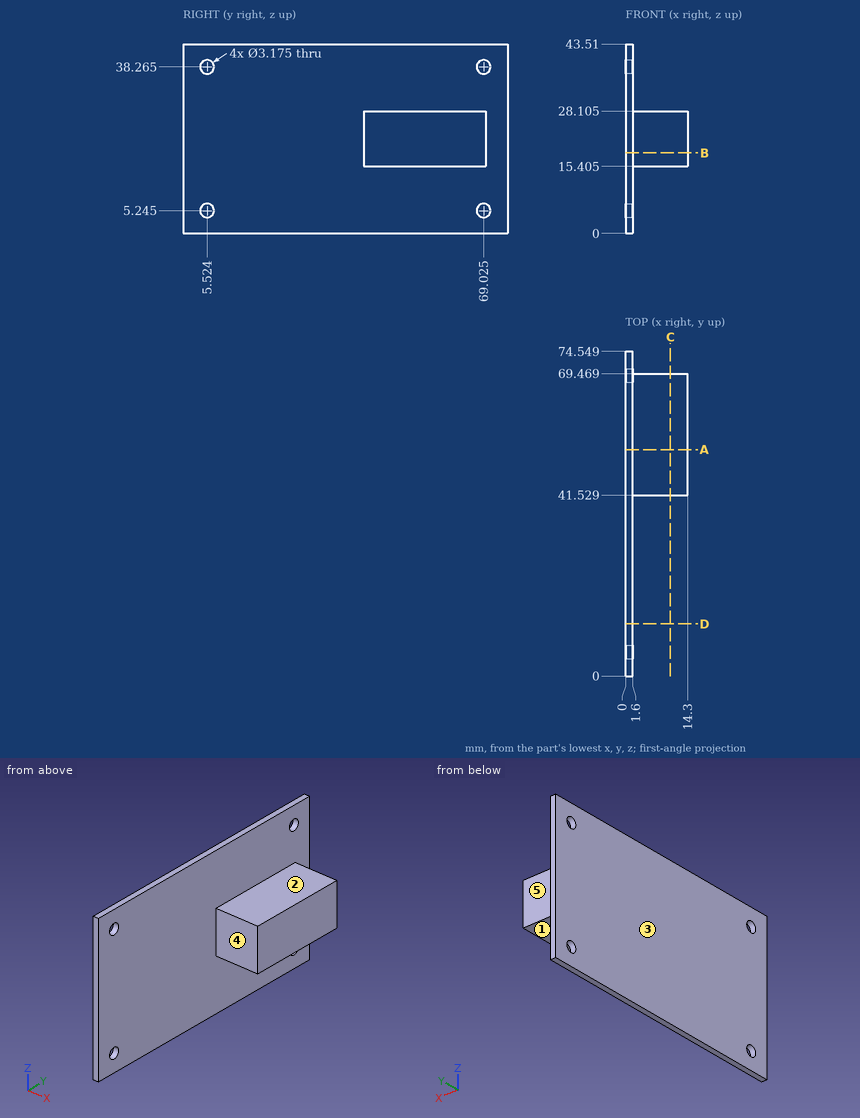
Geometry: see drawing. Coordinates: mm, zero at the bounding-box minimum. A direction names the side the tool comes from. Give positions to 0.01 mm unless a question says otherwise; leave off trailing zeros. Loops run counter-clockwise (first coordinate to the right, second up) from the corner with the lowest first, then second, coordinate; pieces in that order, holes last. Notation, with made-up numbers: M -22,78.25 L -13,78.25 A26 cw -13,111.25 Z; hole C 64,-27.75 d2. An arc over 180 degrees is marked long. Use one line per item in the form item = value.
1. Line query: L1, parallel to X at y = 23.5, z = 23; L2, parallel to Y at x = 9.75, z = 20; L3, parallel to Z at x = 10.5, y = 47.5 (1 decimal). Output: solid intervals per line, ascending.
Numbers:
L1 = 0 to 1.6
L2 = 41.53 to 69.47
L3 = 15.4 to 28.1
2. Section query C-C, the plane x = 10.25. Return the cut outline in (y, z) (1 decimal).
Numbers:
outline = M 41.5,15.4 L 69.5,15.4 L 69.5,28.1 L 41.5,28.1 Z
3. Section query D-D, the plane y = 12. Return the cut outline in (x, z).
Numbers:
outline = M 0,0 L 1.6,0 L 1.6,43.51 L 0,43.51 Z
4. First-contact query: pin 1 (5 mm diameter, centred on y = 5.52, z = 38.27, fed in from -X); pin 2 (4 mm diameter, centred on x = 6.5, z = 19.5, fed in from -Y); pin 3 (1.5 mm diameter, centred on x = 3, y = 38, fed in from -Z); pin 4 (6.5 mm diameter, centred on x = 5.5, y = 54.5, fed in from -Z) (1 decimal). Flat tips, straight axial feed; report the tip coordinate or a pass-through.
Numbers:
pin_1 = 0
pin_2 = 41.53
pin_3 = through
pin_4 = 15.4
5. Section query B-B, the plane z = 18.5. Return the cut outline in (x, y), and give its area (3 significant figures).
Numbers:
outline = M 0,0 L 1.6,0 L 1.6,41.53 L 14.3,41.53 L 14.3,69.47 L 1.6,69.47 L 1.6,74.55 L 0,74.55 Z
area = 474 mm²
6. Reachability of the marked faces 1, 2, 3, 4 and 5 from +Z, -Z, +X, -X, +Y, -Y: full face, straight path, thin tool, end or side. Return the list, or none.
Numbers:
face_1 = -Z, +X, +Y, -Y
face_2 = +Z, +X, +Y, -Y
face_3 = +Z, -Z, -X, +Y, -Y
face_4 = +Z, -Z, +X, -Y
face_5 = +Z, -Z, +X, +Y
7. Section query A-A, the plane y = 52. Return the cut outline in (x, z) (1 decimal).
Numbers:
outline = M 0,0 L 1.6,0 L 1.6,15.4 L 14.3,15.4 L 14.3,28.1 L 1.6,28.1 L 1.6,43.5 L 0,43.5 Z
